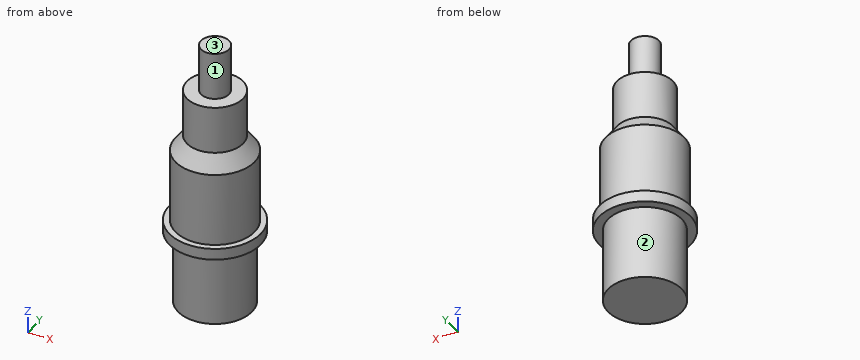
Autodesk Inventor part; units mm, degrees
ref_plane "Work Plane1" through (0, 0, 487.3625) normal (0, 1, 0) x (0, 0, 1)
ref_plane "YZ Plane" through (0, 0, 0) normal (1, 0, 0) x (0, 1, 0)
ref_plane "XZ Plane" through (0, 0, 0) normal (0, 1, 0) x (-1, 0, 0)
sketch "Sketch1" plane through (0, 0, 0) normal (0, 0, 1) x (1, 0, 0)
  circle A0 centre (0, 0) radius 66.675
  dimension "d0" = 133.35
extrude "Extrusion1" add sketch "Sketch1" along normal blind 133.35
sketch "Sketch2" plane through (0, 0, 133.35) normal (0, 0, 1) x (1, 0, 0)
  circle A0 centre (0, 0) radius 82.55
  dimension "d3" = 165.1
extrude "Extrusion2" add sketch "Sketch2" along normal blind 20.6375
sketch "Sketch3" plane through (0, 0, 153.9875) normal (0, 0, 1) x (1, 0, 0)
  circle A0 centre (0, 0) radius 71.4375
  dimension "d6" = 142.875
extrude "Extrusion3" add sketch "Sketch3" along normal blind 133.35
sketch "Sketch4" plane through (0, 0, 287.3375) normal (0, 0, 1) x (1, 0, 0)
  circle A0 centre (0, 0) radius 50.8
  dimension "d9" = 101.6
extrude "Extrusion4" add sketch "Sketch4" along normal blind 114.3
sketch "Sketch5" plane through (0, 0, 401.6375) normal (0, 0, 1) x (1, 0, 0)
  circle A0 centre (0, 0) radius 25.4
  dimension "d12" = 50.8
extrude "Extrusion5" add sketch "Sketch5" along normal blind 85.725
ref_plane "Work Plane1" through (0, 0, 487.3625) normal (0, 1, 0) x (0, 0, 1)
sketch "Sketch6" plane through (0, 0, 487.3625) normal (0, 1, 0) x (0, 0, 1)
  line L0 (-200.025, -71.4375) -> (-200.025, 71.4375)
  line L1 (-171.45, 50.8) -> (-200.025, 71.4375)
  line L2 (-85.725, -50.8) -> (-85.725, 50.8)
  line L3 (-85.725, 50.8) -> (-200.025, 50.8)
  line L4 (-200.025, 71.4375) -> (-200.025, 50.8)
  line L5 (-584.835, 0) -> (97.4725, 0)
  point P0 (-487.3625, 0)
  dimension "d21" = 28.575
revolve "Revolution1" add sketch "Sketch6" angle 360 about axis through (0, 0, 487.3625) along (0, 0, 1) contours L0 L1 L3
properties part number "BC501A _Organic_scintillator_module"
Check sheet for the modelled part. Datum: model origin and axes. Units: mm. Face numbers are marked on the shaded views. A direction names the side the tool comes from. Round coordinates to 2 decimals unless told otherwise and drop trailing zeros. Write each loop counter-clockwise with the first axis right and the second up, starting at its lowest first coordinate (ties: lowest second). Pieces come first, ordered by that corner, then holes. Notation, with made-up numbers: M 70.5,38.25 L 85.5,38.25 A15 cw 85.5,61.25 Z; hole C -38.75,49.5 d2. An arc over 180 degrees is marked long. Write item = value, one per line. Start each with the question number.
1. Tool access check on the marked faces 1, 2 and 3. Record the directions out of +Z, -Z, +X, -X, +Y, -Y that give a thin tool (end or side, any length) a straight path to the whole face; none if there is none.
2. Section check D-D, the plane z = 171.5. Record the cut outline in (x, y) (1 decimal).
3. Section check C-C, the plane z = 411. Record the cut outline in (x, y), then the cut area to 3 significant figures.
4. Gauge pin test, flat ends, axial feed: pin 1 (2 mm diameter, centred on x = -18.5, y = -31.5, fed in from +Z); pin 2 (8 mm diameter, centred on x = 45.5, y = -61, fed in from -Z); pin 3 (8 mm diameter, centred on x = -52, z = 263, fed in from -Y). Record the tip position at first contact, or that the pin passes through.
5. Scan lines: line 1 (Y direction, x = 0.5, z = 136.5); line 2 (Z direction, x = 28.5, y = 32.5); line 3 (Y direction, x = 0, z = 445). Record each from-to range of solid material in increasing order. Write a range as [from, to].
Results found:
q1.face_1 = +Z
q1.face_2 = -Z
q1.face_3 = +Z, +X, -X, +Y, -Y
q2.outline = C 0,0 d142.9
q3.outline = C 0,0 d50.8
q3.area = 2,030 mm^2
q4.pin_1 = 401.64
q4.pin_2 = 133.35
q4.pin_3 = -52.91
q5.line_1 = [-82.55, 82.55]
q5.line_2 = [0, 401.64]
q5.line_3 = [-25.4, 25.4]
